Geometry: final body of the model. Coordinates: model frame, mm. Round coordinates to 2 decimals unless told otherwise and drop trailing zeros. Loops run counter-clockwise (first coordinate to the right, second up) from the corner with the lowest first, then second, coordinate; pieces in that order, holes last. Notation, with made-up numbers: (31, 68.5) - (62, 68.5) arc R20 ccw to (62, 79.5) - close; hole circle Ø3 at (60, -3). An arc over 180 degrees is marked (long way). Answer as CSV lines item,"result".
from build123d import *

# Parameters (mm, degrees)
ESQUISSE1_R             = 140
ESQUISSE1_R_2           = 120
BOSS_EXTRU_1_DEPTH      = 2
ENL_V_MAT_EXTRU_1_REACH = 200
ESQUISSE2_W             = 10
ESQUISSE2_H             = 40
ESQUISSE4_W             = 11.636908411
ESQUISSE4_H             = 60
BOSS_EXTRU_2_DEPTH      = 2
CONG_1_R                = 10
ENL_V_MAT_EXTRU_2_REACH = 200
ESQUISSE5_R             = 1.5


with BuildPart() as part:
    # Esquisse1 → Boss.-Extru.1 (new body)
    with BuildSketch(Plane.XY):
        Circle(ESQUISSE1_R)
        Circle(ESQUISSE1_R_2, mode=Mode.SUBTRACT)
    extrude(amount=BOSS_EXTRU_1_DEPTH)

    # Esquisse2 → Enlèv. mat.-Extru.1 (cut, up to next)
    with BuildSketch(Plane.XY.offset(2), mode=Mode.PRIVATE) as enl_v_mat_extru_1_sk1:
        with Locations((-138, 0)):
            Rectangle(ESQUISSE2_W, ESQUISSE2_H)
    enl_v_mat_extru_1_tool1 = extrude(enl_v_mat_extru_1_sk1.sketch, amount=-ENL_V_MAT_EXTRU_1_REACH, mode=Mode.PRIVATE) & part.part
    add(enl_v_mat_extru_1_tool1.solids().sort_by_distance((-138, 0, 2))[0], mode=Mode.SUBTRACT)

    # Esquisse4 → Boss.-Extru.2 (add)
    with BuildSketch(Plane.XY.offset(2)):
        with Locations((-127.181545795, 10)):
            Rectangle(ESQUISSE4_W, ESQUISSE4_H)
    extrude(amount=-BOSS_EXTRU_2_DEPTH)

    # Congé1
    # the kernel refuses this fillet: 10 mm, written as the material it adds along each edge
    with BuildSketch(Plane(origin=(-133, -20, 2), x_dir=(-1, 0, 0), z_dir=(0, 0, -1))) as cong_1_piece_1:
        with BuildLine():
            CenterArc((10, 8.962280802), CONG_1_R, 180, 63.666611113)
            Line((0, 8.962280802), (-0.2, 8.962280802))
            Line((-0.2, 8.962280802), (-0.2, 0))
            Line((-0.2, 0), (0, -0.2))
            ThreePointArc((0, -0.2), (2.782032303, -0.2), (5.475345898, -0.179245616))
            Line((5.475345898, -0.179245616), (5.564064606, 0))
        make_face()
    extrude(amount=2)
    with BuildSketch(Plane(origin=(-133, 20, 2), x_dir=(-1, 0, 0), z_dir=(0, 0, -1))) as cong_1_piece_2:
        with BuildLine():
            CenterArc((10, -8.962280802), CONG_1_R, 116.333388887, 63.666611113)
            Line((0, -8.962280802), (-0.2, -8.962280802))
            Line((-0.2, -8.962280802), (-0.2, 0))
            Line((-0.2, 0), (0, 0.2))
            ThreePointArc((0, 0.2), (2.782032303, 0.2), (5.475345898, 0.179245616))
            Line((5.475345898, 0.179245616), (5.564064606, 0))
        make_face()
    extrude(amount=2)

    # Esquisse5 → Enlèv. mat.-Extru.2 (cut, up to next)
    with BuildSketch(Plane.XY.offset(2), mode=Mode.PRIVATE) as enl_v_mat_extru_2_sk1:
        with Locations((-35.199390134, -131.365912375)):
            Circle(ESQUISSE5_R)
    enl_v_mat_extru_2_tool1 = extrude(enl_v_mat_extru_2_sk1.sketch, amount=-ENL_V_MAT_EXTRU_2_REACH, mode=Mode.PRIVATE) & part.part
    # Esquisse5 → Enlèv. mat.-Extru.2 (cut, up to next)
    with BuildSketch(Plane.XY.offset(2), mode=Mode.PRIVATE) as enl_v_mat_extru_2_sk2:
        with Locations((35.199390134, -131.365912375)):
            Circle(ESQUISSE5_R)
    enl_v_mat_extru_2_tool2 = extrude(enl_v_mat_extru_2_sk2.sketch, amount=-ENL_V_MAT_EXTRU_2_REACH, mode=Mode.PRIVATE) & part.part
    # Esquisse5 → Enlèv. mat.-Extru.2 (cut, up to next)
    with BuildSketch(Plane.XY.offset(2), mode=Mode.PRIVATE) as enl_v_mat_extru_2_sk3:
        with Locations((-35.199390134, 131.365912375)):
            Circle(ESQUISSE5_R)
    enl_v_mat_extru_2_tool3 = extrude(enl_v_mat_extru_2_sk3.sketch, amount=-ENL_V_MAT_EXTRU_2_REACH, mode=Mode.PRIVATE) & part.part
    # Esquisse5 → Enlèv. mat.-Extru.2 (cut, up to next)
    with BuildSketch(Plane.XY.offset(2), mode=Mode.PRIVATE) as enl_v_mat_extru_2_sk4:
        with Locations((35.199390134, 131.365912375)):
            Circle(ESQUISSE5_R)
    enl_v_mat_extru_2_tool4 = extrude(enl_v_mat_extru_2_sk4.sketch, amount=-ENL_V_MAT_EXTRU_2_REACH, mode=Mode.PRIVATE) & part.part
    add(enl_v_mat_extru_2_tool1.solids().sort_by_distance((-35.19939, -131.365912, 2))[0], mode=Mode.SUBTRACT)
    add(enl_v_mat_extru_2_tool2.solids().sort_by_distance((35.19939, -131.365912, 2))[0], mode=Mode.SUBTRACT)
    add(enl_v_mat_extru_2_tool3.solids().sort_by_distance((-35.19939, 131.365912, 2))[0], mode=Mode.SUBTRACT)
    add(enl_v_mat_extru_2_tool4.solids().sort_by_distance((35.19939, 131.365912, 2))[0], mode=Mode.SUBTRACT)


solid = part.part
(1) Section A-A (y = 0). Output: boundary loops of the cut face in (x, z).
Findings below:
outline,"(-133, 0) - (-120, 0) - (-120, 2) - (-133, 2) - close; (120, 0) - (140, 0) - (140, 2) - (120, 2) - close"
(2) Section C-C (z = 0.95). Output: boundary loops of the cut face in (x, y).
Findings below:
outline,"(-138.56, -20) arc R140 ccw (long way) to (-138.56, 20) arc R10 cw to (-133, 11.04) - (-133, -11.04) arc R10 cw to start; hole circle Ø240 at (0, 0); hole circle Ø3 at (-35.2, -131.37); hole circle Ø3 at (-35.2, 131.37); hole circle Ø3 at (35.2, -131.37); hole circle Ø3 at (35.2, 131.37)"
(3) Draft query along X for faces 1 (the face through (103, 63, 0)), 2 (the face through (-119.884, 5.276, 0.986)), 3 (the face through (139.877, -5.875, 0.986)). Return one class per face: pulls with the +X half, pulls with the -X half, needs draft (parallel to the pull), parting line crosses it, or undercut.
Findings below:
face 1,"needs draft"
face 2,"undercut"
face 3,"parting line crosses it"
(4) Material intervals for line 1 along Y through (x, z) = (34.5, 0.5); line 2 along X through (y, z) = (-2, 0.3); line 3 along Y through (x, z) = (0, 1.35), sorted ascending.
Findings below:
line 1,"-135.68 to -132.69, -130.04 to -114.93, 114.93 to 130.04, 132.69 to 135.68"
line 2,"-133 to -119.98, 119.98 to 139.99"
line 3,"-140 to -120, 120 to 140"
(5) Section B-B (x = 0). Output: boundary loops of the cut face in (y, z).
Findings below:
outline,"(-140, 0) - (-120, 0) - (-120, 2) - (-140, 2) - close; (120, 0) - (140, 0) - (140, 2) - (120, 2) - close"
